from build123d import *

# Parameters (mm, degrees)
SKETCH1_W           = 17
SKETCH1_H           = 20
SKETCH1_R           = 1.5
BOSS_EXTRUDE1_DEPTH = 7
SKETCH2_R           = 1.5
CUT_EXTRUDE6_DEPTH  = 2.6


with BuildPart() as part:
    # Sketch1 → Boss-Extrude1 (new body)
    with BuildSketch(Plane(origin=(0, 0, 0), x_dir=(1, 0, 0), z_dir=(0, 1, 0))):
        with Locations((-3.5, -5)):
            Rectangle(SKETCH1_W, SKETCH1_H)
        Circle(SKETCH1_R, mode=Mode.SUBTRACT)
        with Locations((-7, -10)):
            Circle(SKETCH1_R, mode=Mode.SUBTRACT)
        with Locations((-7, 0)):
            Circle(SKETCH1_R, mode=Mode.SUBTRACT)
        with Locations((0, -10)):
            Circle(SKETCH1_R, mode=Mode.SUBTRACT)
    extrude(amount=BOSS_EXTRUDE1_DEPTH)

    # Sketch2 → Cut-Extrude6 (cut)
    with BuildSketch(Plane(origin=(0, 7, 0), x_dir=(1, 0, 0), z_dir=(0, 1, 0))):
        with BuildLine():
            Line((-7, -13.75), (0, -13.75))
            ThreePointArc((0, -13.75), (3.75, -10), (0, -6.25))
            Line((0, -6.25), (-7, -6.25))
            ThreePointArc((-7, -6.25), (-10.75, -10), (-7, -13.75))
        make_face()
        with Locations((-7, -10)):
            Circle(SKETCH2_R, mode=Mode.SUBTRACT)
        with Locations((0, -10)):
            Circle(SKETCH2_R, mode=Mode.SUBTRACT)
        with BuildLine():
            ThreePointArc((-7, 3.75), (-10.75, 0), (-7, -3.75))
            Line((-7, -3.75), (0, -3.75))
            ThreePointArc((0, -3.75), (3.75, 0), (0, 3.75))
            Line((0, 3.75), (-7, 3.75))
        make_face()
        with Locations((-7, 0)):
            Circle(SKETCH2_R, mode=Mode.SUBTRACT)
        Circle(SKETCH2_R, mode=Mode.SUBTRACT)
    extrude(amount=-CUT_EXTRUDE6_DEPTH, mode=Mode.SUBTRACT)


solid = part.part
The model under review builds one solid part; all positions refer to its coordinate system, in mm. A direction names the side the tool comes from. Give positions to 0.01 mm unless a question says otherwise; leave off trailing zeros. Order: outer loops, then holes, each group sorted by start corner. A loop starts at its lowest first (then second) coordinate and runs counter-clockwise, first axis right, second up. Notation, with made-up numbers: M 84,-40 L 114,-40 A27 cw 114,-16 Z; hole C 22.25,68.25 d6. An arc over 180 degrees is marked long. Use one line per item in the form item = value. Start each with the question number.
Item 1: We need section D-D on y = 3.5. Give the boundary of the cut face in (x, z), plus the area to 3 significant figures.
Item 2: We need section B-B on y = 6.75. Give the boundary of the cut face in (x, z).
Item 3: We need section A-A on z = 0. Give the boundary of the cut face in (x, y).
Item 4: The part is to be moulded in two halves that separate along Z. For faces 3 (the flat face through (-4, 7, 5)), 4 (the flat face through (-4, 3, -5)), 5 (the cylindrical face through (-8.2, 2.2, 10.9)), 6 (the flat face through (-4, 4.4, 10)), say which applies: pulls with the +Z half, pulls with the -Z half, needs draft (parallel to the pull), parting line crosses it, or undercut.
Item 5: To check wall thickness, follow line 1 along Z through (x, y) = (0, 2.55); line 2 along X through (y, z) = (2.15, 0); line 3 along X through (y, z) = (3.5, 11). State the ranges of each line that lie inside material, in increasing order. Write a range as from..to.
Item 6: For faces 1 (the cylindrical face through (3.75, 5.72, 0.08)), 2 (the flat face through (-12, 3, 5)), list the 3-axis set-ups (+Z, -Z, +X, -X, +Y, -Y) from which the entire face can be reached by the end or side of a thin tool; tool diameter is ignored.
Item 7: We need section C-C on x = -8.25. Give the boundary of the cut face in (y, z).
Item 8: Insertion check: pin 1 Ø4 at (x, z) = (-6.5, 9.5) entering from +Y. The pin has a flat end and moves straight along its axis. Give the tip position at first contact, or say it passes through.
Completed:
q1.outline = M -12,-5 L 5,-5 L 5,15 L -12,15 Z; hole C -7,0 d3; hole C -7,10 d3; hole C 0,0 d3; hole C 0,10 d3
q1.area = 312 mm²
q2.outline = M -12,-5 L 5,-5 L 5,15 L -12,15 Z; hole M -7,-3.75 L 0,-3.75 A3.75 ccw 0,3.75 L -7,3.75 A3.75 ccw Z; hole M -7,6.25 L 0,6.25 A3.75 ccw 0,13.75 L -7,13.75 A3.75 ccw Z
q3.outline = M -12,0 L -8.5,0 L -8.5,4.4 L -10.75,4.4 L -10.75,7 L -12,7 Z; M -5.5,0 L -1.5,0 L -1.5,4.4 L -5.5,4.4 Z; M 1.5,0 L 5,0 L 5,7 L 3.75,7 L 3.75,4.4 L 1.5,4.4 Z
q4.face_3 = needs draft
q4.face_4 = pulls with the -Z half
q4.face_5 = undercut
q4.face_6 = undercut
q5.line_1 = -5..-1.5, 1.5..8.5, 11.5..15
q5.line_2 = -12..-8.5, -5.5..-1.5, 1.5..5
q5.line_3 = -12..-8.12, -5.88..-1.12, 1.12..5
q6.face_1 = +Y
q6.face_2 = +Z, -Z, -X, +Y, -Y
q7.outline = M 0,-5 L 7,-5 L 7,-3.54 L 4.4,-3.54 L 4.4,-0.83 L 0,-0.83 Z; M 0,0.83 L 4.4,0.83 L 4.4,3.54 L 7,3.54 L 7,6.46 L 4.4,6.46 L 4.4,9.17 L 0,9.17 Z; M 0,10.83 L 4.4,10.83 L 4.4,13.54 L 7,13.54 L 7,15 L 0,15 Z
q8.pin_1 = 4.4
